The model under review builds one solid part; all positions refer to its coordinate system, in mm. Face numbers are marked on the shaded views. A direction names the side the tool comes from. Round coordinates to 2 decimals unless told otherwise and drop trailing zeros. Write each loop counter-clockwise with the first axis right and the second up, starting at its lowest first coordinate (ties: lowest second). Pieces come first, ordered by that corner, then holes. Notation, with made-up numbers: (79, 36) - (118, 36) arc R23 cw to (118, 61) - close; hole circle Ø10 at (-3, 43). An arc over 180 degrees is marked (long way). Use one line per item in the form item = value.
from build123d import *

# Parameters (mm, degrees)
CHAMFER_1_SIZE = 1
FILLET_1_R     = 0.4


with BuildPart() as part:
    # 스케치1 → 회전1 (revolve)
    with BuildSketch(Plane(origin=(0, 0, 0), x_dir=(1, 0, 0), z_dir=(0, 1, 0))):
        with BuildLine():
            Line((0, 0), (4, 0))
            Line((4, 0), (5.894700279, 0.5))
            Line((5.894700279, 0.5), (10, 0.5))
            Line((10, 0.5), (10, -4.75))
            Line((10, -4.75), (9.37, -4.75))
            ThreePointArc((9.37, -4.75), (8.62, -5.5), (9.37, -6.25))
            Line((9.37, -6.25), (10, -6.25))
            Line((10, -6.25), (10, -11.5))
            Line((10, -11.5), (7.2, -11.5))
            Line((7.2, -11.5), (7, -2.5))
            Line((7, -2.5), (0, -2.5))
            Line((0, -2.5), (0, 0))
        make_face()
    revolve(axis=Axis((0, 0, 2.5), (0, 0, -1)))

    # 모따기1
    chamfer_1_edges = [part.edges().sort_by_distance(p)[0] for p in [
        (-10, 0, 11.5),
        (-10, 0, -0.5),
    ]]
    chamfer(chamfer_1_edges, length=CHAMFER_1_SIZE)

    # 필렛1
    fillet_1_edges = [part.edges().sort_by_distance(p)[0] for p in [
        (-7.2, 0, 11.5),
        (-5.894700279, 0, -0.5),
    ]]
    fillet(fillet_1_edges, radius=FILLET_1_R)


solid = part.part
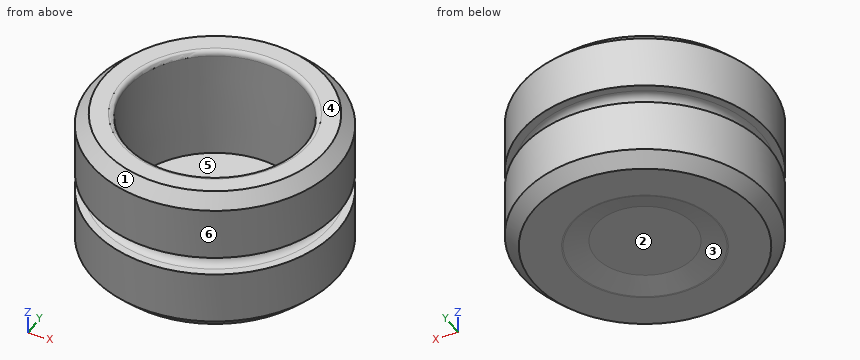
(1) Add section D-D on z = 4.5. Write out the cut boundary in (x, y), then the cut area to 3 significant figures.
Geometry results:
outline = circle Ø20 at (0, 0); hole circle Ø14.09 at (0, 0)
area = 158 mm2
(2) Machinability: for the marked faces 5 and 6, which of the approach directions +Z, -Z, +X, -X, +Y, -Y give a long, thin tool a straight path to every point of the face, cutting with its end or side? Answer none if there is none.
Geometry results:
face_5 = +Z
face_6 = +Z, -Z
(3) To check wall thickness, follow L1, parallel to X at y = -1, z = 9; L2, parallel to Z at x = -6.25, y = 3; L3, parallel to X at y = -5.5, z = 9.75. State the ranges of each line that lie inside material, in increasing order.
Geometry results:
L1 = -9.95 to -7.07, 7.07 to 9.95
L2 = -0.5 to 2.5
L3 = -8.35 to -4.59, 4.59 to 8.35
(4) Add section C-C on z = 8.25. Write out the cut boundary in (x, y).
Geometry results:
outline = circle Ø20 at (0, 0); hole circle Ø14.26 at (0, 0)
(5) The part is to be moulded in two halves that separate along X. For the marked faces 1, 2, 3 and 4, say which applies: +X half, -X half, draft (parallel to the pull), parting line (faces both ways), or undercut.
Geometry results:
face_1 = parting line
face_2 = undercut
face_3 = undercut
face_4 = draft
(6) Insertion check: P1, Ø4, axis at y = -4.5, z = 5, coming from the +X side. The pin has a flat end and moves straight along its axis. Give the tip position at first contact, or say it passes through.
Geometry results:
P1 = 9.68
(7) Add section A-A on x = 0. Write out the cut boundary in (y, z).
Geometry results:
outline = (-10, 0.5) - (-9, -0.5) - (-5.95, -0.5) arc R0.4 ccw to (-5.84, -0.49) - (-4, 0) - (4, 0) - (5.84, -0.49) arc R0.4 ccw to (5.95, -0.5) - (9, -0.5) - (10, 0.5) - (10, 4.75) - (9.37, 4.75) arc R0.75 cw to (9.37, 6.25) - (10, 6.25) - (10, 10.5) - (9, 11.5) - (7.59, 11.5) arc R0.4 ccw to (7.19, 11.11) - (7, 2.5) - (-7, 2.5) - (-7.19, 11.11) arc R0.4 ccw to (-7.59, 11.5) - (-9, 11.5) - (-10, 10.5) - (-10, 6.25) - (-9.37, 6.25) arc R0.75 cw to (-9.37, 4.75) - (-10, 4.75) - close
